The drawing under review shows one solid part. Ordinate dimensions are in mm from its lowest x, y, z. Coordinates: 2 decimals unless noted, no trailing zeros. Order: outer loops, then holes, each group sorted by start corner. A loop starts at its lowest first (then second) coordinate and runs counter-clockwise, first axis right, second up. Notation, with made-up numbers: M 74.5,-33.75 L 132.5,-33.75 A21 cw 132.5,-25.75 Z; hole C 60.5,-32 d9. An arc over 180 degrees is marked long. Answer as a JSON object with one key per item and string values.
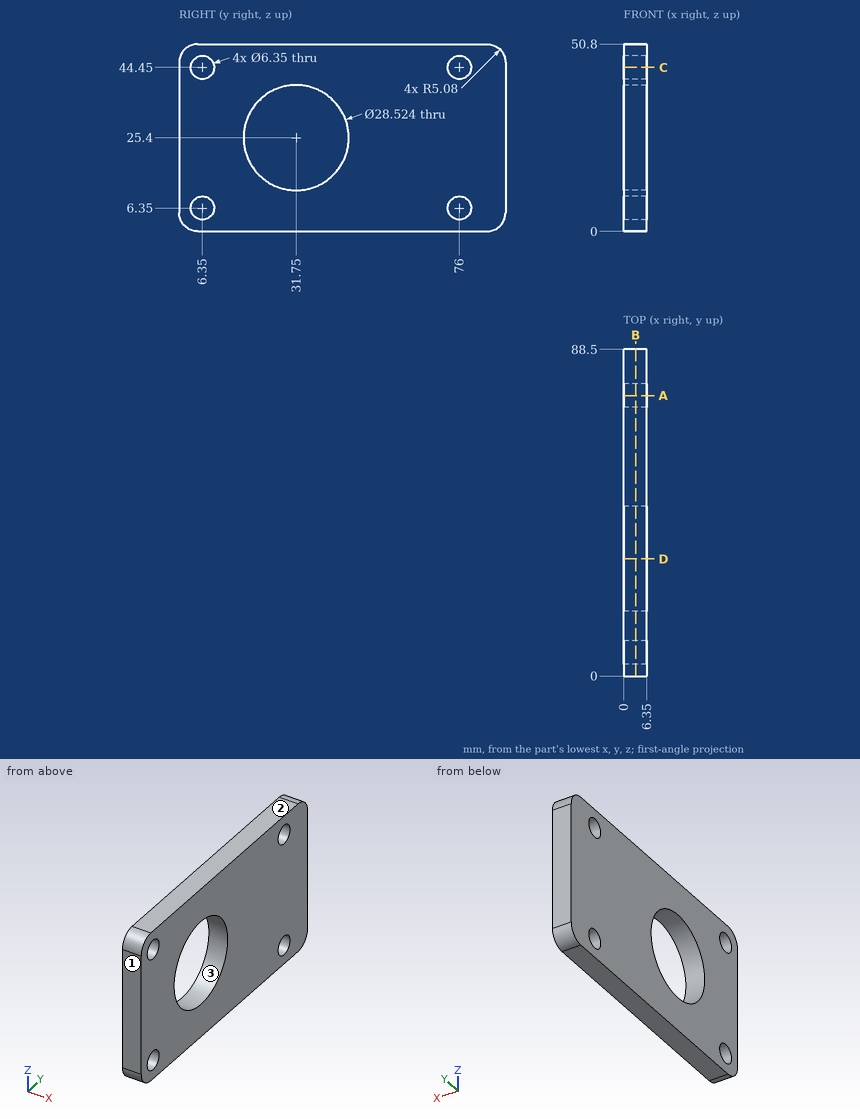
1) Add section B-B (x = 3.25). Count the separate pieces of the cut face and the enclosed holes in it, and give its area (3 significant figures).
Taken from the geometry:
{"separate pieces": "1", "enclosed holes": "5", "area": "3,710 mm2"}
2) Add section C-C (z = 44.45). State the section outline as (x, y) points (3 decimals), and give its area (3 significant figures).
Taken from the geometry:
{"outline": "M 0,0 L 6.35,0 L 6.35,3.175 L 0,3.175 Z; M 0,9.525 L 6.35,9.525 L 6.35,72.825 L 0,72.825 Z; M 0,79.175 L 6.35,79.175 L 6.35,88.5 L 0,88.5 Z", "area": "481 mm2"}
3) Add section A-A (y = 76). State the section outline as (x, z) points (3 decimals).
Taken from the geometry:
{"outline": "M 0,0 L 6.35,0 L 6.35,3.175 L 0,3.175 Z; M 0,9.525 L 6.35,9.525 L 6.35,41.275 L 0,41.275 Z; M 0,47.625 L 6.35,47.625 L 6.35,50.8 L 0,50.8 Z"}
4) Add section D-D (y = 31.75). State the section outline as (x, z) points, and give its area (3 significant figures).
Taken from the geometry:
{"outline": "M 0,0 L 6.35,0 L 6.35,11.14 L 0,11.14 Z; M 0,39.66 L 6.35,39.66 L 6.35,50.8 L 0,50.8 Z", "area": "141 mm2"}
5) Mouldability with a two-part tool opening along Y and no side actions: class the marked faces 1, 2 and 3 as released by +Y, released by -Y, zero draft, split by the parting line, or undercut.
Taken from the geometry:
{"face 1": "released by -Y", "face 2": "zero draft", "face 3": "undercut"}
6) To check wall thickness, follow L1, parallel to Y at x = 5.25, z = 44.45 (3 decimals); L2, parallel to Y at x = 1, z = 45; L3, parallel to Z at x = 1.75, y = 4 (1 decimal). State the ranges of each line that lie inside material, in increasing order.
Taken from the geometry:
{"L1": "y = 0 to 3.175, 9.525 to 72.825, 79.175 to 88.5", "L2": "y = 0 to 3.22, 9.48 to 72.87, 79.13 to 88.5", "L3": "z = 0.1 to 4.2, 8.5 to 42.3, 46.6 to 50.7"}
